CAD build for the part. Positions are in the model's coordinates, mm. Face numbers are marked on the shaded views. Give positions to 0.01 mm unless a question says otherwise; leave off trailing zeros. Loops run counter-clockwise (first coordinate to the right, second up) from the corner with the lowest first, then second, coordinate; pieces in that order, holes last.
```python
from build123d import *

# Parameters (mm, degrees)
SKETCH1_W                = 66.35
SKETCH1_H                = 69.18
SKETCH1_R                = 29
BOSS_EXTRUDE1_DEPTH      = 7
SKETCH3_W                = 66.35
SKETCH3_H                = 69.18
SKETCH3_R                = 32.25
BOSS_EXTRUDE2_DEPTH      = 6
CUT_EXTRUDE1_DEPTH       = 3.18
CUT_EXTRUDE5_DEPTH       = 1.25
M3_CLEARANCE_HOLE3_D     = 3.2
M3_CLEARANCE_HOLE3_DEPTH = 10
M3_CLEARANCE_HOLE3_TIP   = 0.96137699
SKETCH14_R               = 3
CUT_EXTRUDE3_DEPTH       = 11
CUT_EXTRUDE4_DEPTH       = 1.25
M3_CLEARANCE_HOLE2_D     = 3.2
FILLET1_R                = 1


with BuildPart() as part:
    # Sketch1 → Boss-Extrude1 (new body)
    with BuildSketch(Plane(origin=(0, 0, 0), x_dir=(0, 0, -1), z_dir=(1, 0, 0))):
        Rectangle(SKETCH1_W, SKETCH1_H)
        with Locations((0, 1.91)):
            Circle(SKETCH1_R, mode=Mode.SUBTRACT)
    extrude(amount=BOSS_EXTRUDE1_DEPTH)

    # Sketch3 → Boss-Extrude2 (add)
    with BuildSketch(Plane(origin=(7, 0, 0), x_dir=(0, 0, -1), z_dir=(1, 0, 0))):
        Rectangle(SKETCH3_W, SKETCH3_H)
        with Locations((0, 1.91)):
            Circle(SKETCH3_R, mode=Mode.SUBTRACT)
    extrude(amount=BOSS_EXTRUDE2_DEPTH)

    # Sketch5 → Cut-Extrude1 (cut)
    with BuildSketch(Plane(origin=(0, 34.59, 0), x_dir=(1, 0, 0), z_dir=(0, 1, 0))):
        Polygon((3.175, 33.175), (11.175, 33.175), (11.175, 25.175), (3.175, 25.175), (3.175, -25.175), (11.175, -25.175), (11.175, -33.175), (3.175, -33.175), (0, -33.175), (0, 33.175), align=None)
    extrude(amount=-CUT_EXTRUDE1_DEPTH, mode=Mode.SUBTRACT)

    # Sketch8 → Cut-Extrude5 (cut, symmetric)
    with BuildSketch(Plane(origin=(0, 28.41, 0), x_dir=(1, 0, 0), z_dir=(0, 1, 0))):
        Polygon((4.425, -30.76271324), (4.425, -33.175), (9.925, -33.175), (9.925, -30.76271324), (9.925, -27.58728676), (7.175, -25.999573519), (4.425, -27.58728676), align=None)
        Polygon((4.425, 30.76271324), (4.425, 27.58728676), (7.175, 25.999573519), (9.925, 27.58728676), (9.925, 30.76271324), (9.925, 33.175), (4.425, 33.175), align=None)
    extrude(amount=CUT_EXTRUDE5_DEPTH, both=True, mode=Mode.SUBTRACT)

    # M3 Clearance Hole3
    with Locations(Plane(origin=(0, 31.41, 0), x_dir=(1, 0, 0), z_dir=(0, 1, 0))):
        with Locations((7.175, 29.175), (7.175, -29.175)):
            Hole(M3_CLEARANCE_HOLE3_D / 2, depth=M3_CLEARANCE_HOLE3_DEPTH)
            with Locations((0, 0, -(M3_CLEARANCE_HOLE3_DEPTH + M3_CLEARANCE_HOLE3_TIP / 2))):  # 118° drill point
                Cone(0, M3_CLEARANCE_HOLE3_D / 2, M3_CLEARANCE_HOLE3_TIP, mode=Mode.SUBTRACT)

    # Sketch14 → Cut-Extrude3 (cut)
    with BuildSketch(Plane(origin=(13, 0, 0), x_dir=(0, 0, -1), z_dir=(1, 0, 0))):
        with Locations(Location((0, -31.09, 0), (0, 0, 17.014495586))):
            Circle(SKETCH14_R)
    extrude(amount=-CUT_EXTRUDE3_DEPTH, mode=Mode.SUBTRACT)

    # Sketch15 → Cut-Extrude4 (cut, symmetric)
    with BuildSketch(Plane(origin=(10, 0, 0), x_dir=(0, 0, -1), z_dir=(1, 0, 0))):
        Polygon((19.75, -27.67771324), (19.75, -34.59), (25.25, -34.59), (25.25, -27.67771324), (25.25, -24.50228676), (22.5, -22.914573519), (19.75, -24.50228676), align=None)
        Polygon((-25.25, 31.49771324), (-25.25, 28.32228676), (-22.5, 26.734573519), (-19.75, 28.32228676), (-19.75, 31.49771324), (-19.75, 34.59), (-25.25, 34.59), align=None)
    extrude(amount=CUT_EXTRUDE4_DEPTH, both=True, mode=Mode.SUBTRACT)

    # M3 Clearance Hole2 (through all)
    with Locations(Plane(origin=(13, 0, 0), x_dir=(0, 0, -1), z_dir=(1, 0, 0))):
        with Locations((0, -31.09), (-22.5, 29.91), (22.5, -26.09)):
            Hole(M3_CLEARANCE_HOLE2_D / 2)

    # Fillet1
    # the kernel refuses this fillet: 1 mm, written as the material it takes off along each edge
    with BuildSketch(Plane(origin=(15.541447309, -30.212159091, -2.86869227), x_dir=(0, 0.10463908586340893, -0.9945102622445231), z_dir=(-1, 0, 0))) as fillet1_piece_1:
        with BuildLine():
            CenterArc((1.032339837, 0.999875789), FILLET1_R, 186.128452326, 82.968476456)
            ThreePointArc((0.038054785, 0.893117956), (0.052480052, 0.445133596), (0, 0))
            ThreePointArc((0, 0), (0.508289462, 0.004005802), (1.016578924, 0))
        make_face()
    extrude(amount=8.541447309, mode=Mode.SUBTRACT)
    with BuildSketch(Plane(origin=(15.541447309, -30.212159091, 2.86869227), x_dir=(0, 0.10463908586340893, 0.9945102622445231), z_dir=(-1, 0, 0))) as fillet1_piece_2:
        with BuildLine():
            CenterArc((1.032339837, -0.999875789), FILLET1_R, 90.903071218, 82.968476456)
            ThreePointArc((0.038054785, -0.893117956), (0.052480052, -0.445133596), (0, 0))
            ThreePointArc((0, 0), (0.508289462, -0.004005802), (1.016578924, 0))
        make_face()
    extrude(amount=8.541447309, mode=Mode.SUBTRACT)
    with BuildSketch(Plane(origin=(3.175, 37.09, -25.175), x_dir=(1, 0, 0), z_dir=(0, -1, 0)), Plane(origin=(3.175, 37.09, 25.175), x_dir=(0, 0, -1), z_dir=(0, -1, 0))) as fillet1_piece_3:
        with BuildLine():
            CenterArc((FILLET1_R, FILLET1_R), FILLET1_R, 180, 90)
            Line((0, FILLET1_R), (0, 0))
            Line((0, 0), (FILLET1_R, 0))
        make_face()
    extrude(amount=5.68, mode=Mode.SUBTRACT)
    with BuildSketch(Plane(origin=(11.175, 31.41, -33.175), x_dir=(0, -1, 0), z_dir=(-1, 0, 0)), Plane(origin=(-2.5, 31.41, 33.175), x_dir=(0, -1, 0), z_dir=(1, 0, 0))) as fillet1_piece_4:
        with BuildLine():
            CenterArc((FILLET1_R, FILLET1_R), FILLET1_R, 180, 90)
            Line((0, FILLET1_R), (0, 0))
            Line((0, 0), (FILLET1_R, 0))
        make_face()
    extrude(amount=13.675, mode=Mode.SUBTRACT)
    with BuildSketch(Plane(origin=(-2.5, -34.59, -33.175), x_dir=(0, 0, 1), z_dir=(1, 0, 0)), Plane(origin=(15.5, -34.59, 33.175), x_dir=(0, 0, -1), z_dir=(-1, 0, 0))) as fillet1_piece_5:
        with BuildLine():
            CenterArc((FILLET1_R, -FILLET1_R), FILLET1_R, 90, 90)
            Line((0, -FILLET1_R), (0, 0))
            Line((0, 0), (FILLET1_R, 0))
        make_face()
    extrude(amount=18, mode=Mode.SUBTRACT)
    with BuildSketch(Plane(origin=(15.5, 34.59, 33.175), x_dir=(0, -1, 0), z_dir=(-1, 0, 0)), Plane(origin=(8.675, 34.59, -33.175), x_dir=(0, -1, 0), z_dir=(1, 0, 0))) as fillet1_piece_6:
        with BuildLine():
            CenterArc((FILLET1_R, -FILLET1_R), FILLET1_R, 90, 90)
            Line((0, -FILLET1_R), (0, 0))
            Line((0, 0), (FILLET1_R, 0))
        make_face()
    extrude(amount=6.825, mode=Mode.SUBTRACT)


solid = part.part
```
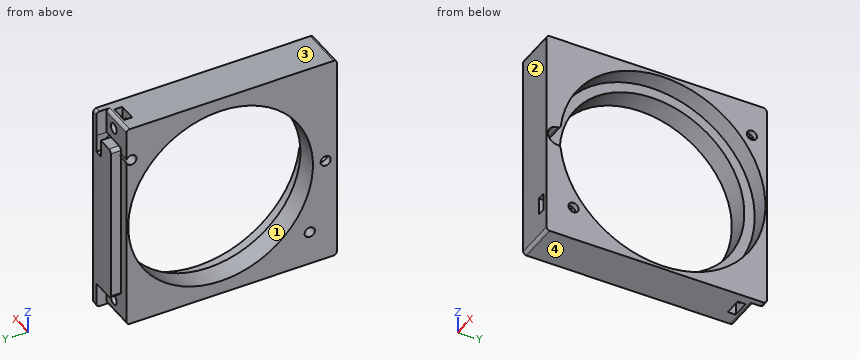
1. Drop flat-ended pins along their axis: pin 1 (2.5 mm diameter, centred on x = 7, y = 32.5, fed in from +Z); pin 2 (0.8 mm diameter, centred on x = 10, y = 31, fed in from +Z); pin 3 (5 mm diameter, centred on y = -31, z = 0, fed in from +X). Give the stop position or say it passes through.
Responses:
pin 1: stops at z = 32.72
pin 2: stops at z = 33.16
pin 3: stops at x = 2
2. Pull direction Z, two halves, no side cores. Call the marked faces 1, 2, 3 and 4: released by +Z, released by -Z, zero draft, split by the parting line, or undercut.
Responses:
face 1: undercut
face 2: zero draft
face 3: released by +Z
face 4: released by -Z
3. Saw through at A-A, the plane z = 0. List the corners of the cut face in (x, y) (3 decimals).
Responses:
outline: (0, -34.59) - (13, -34.59) - (13, -34.09) - (2, -34.09) - (2, -32.69) - (0, -32.69) - close; (0, -29.49) - (2, -29.49) - (2, -28.09) - (7, -28.09) - (7, -27.09) - (0, -27.09) - close; (0, 30.91) - (7, 30.91) - (7, 34.16) - (13, 34.16) - (13, 34.59) - (3.175, 34.59) - (3.175, 31.41) - (0, 31.41) - close
4. Saw through at B-B, the plane y = -14.5. List the corners of the cut face in (x, z) (1 decimal), and give its area (3 significant figures).
Responses:
outline: (0, -33.2) - (13, -33.2) - (13, -27.8) - (7, -27.8) - (7, -23.9) - (0, -23.9) - close; (0, 23.9) - (7, 23.9) - (7, 27.8) - (13, 27.8) - (13, 33.2) - (0, 33.2) - close
area: 195 mm2
5. Probe line 1 along Y through (x, z) = (0.9, 0); line 2 along Y through (x, z) = (5, -1); line 3 along Y through (x, z) = (9.75, 17.5). List the from-to ranges inside material, lowest first.
Responses:
line 1: y = -34.59 to -32.69, -29.49 to -27.09, 30.91 to 31.41
line 2: y = -34.59 to -33.92, -28.26 to -27.07, 30.89 to 34.59
line 3: y = -34.59 to -25.18, 29 to 34.59
6. Saw through at D-D, the plane z = -12.5. List the corners of the cut face in (x, y) (3 decimals), and give its area (3 significant figures).
Responses:
outline: (0, -34.59) - (13, -34.59) - (13, -27.819) - (7, -27.819) - (7, -24.258) - (0, -24.258) - close; (0, 28.078) - (7, 28.078) - (7, 31.639) - (13, 31.639) - (13, 34.59) - (3.175, 34.59) - (3.175, 31.41) - (0, 31.41) - close
area: 166 mm2
7. Saw through at C-C, the plane y = -26.09. List the corners of the cut face in (x, z) (3 decimals), and give its area (3 significant figures).
Responses:
outline: (0, -33.175) - (13, -33.175) - (13, -24.1) - (11.25, -24.1) - (11.25, -25.25) - (8.75, -25.25) - (8.75, -24.1) - (0, -24.1) - close; (0, -20.9) - (8.75, -20.9) - (8.75, -19.75) - (11.25, -19.75) - (11.25, -20.9) - (13, -20.9) - (13, -16.002) - (7, -16.002) - (7, -7.55) - (0, -7.55) - close; (0, 7.55) - (7, 7.55) - (7, 16.002) - (13, 16.002) - (13, 33.175) - (0, 33.175) - close
area: 517 mm2
